Verification items for the finished model (mm, model axes). A direction names the side the tool comes from. Give positions to 0.01 mm unless a question says otherwise; leave off trailing zeros. Order: outer loops, then holes, each group sorted by start corner. A loop starts at its lowest first (then second) coordinate and runs counter-clockwise, first axis right, second up. Notation, with made-up numbers: M -26,12.25 L 3,12.25 A20 cw 3,50.25 Z; hole C 26,84 d1. An arc over 180 degrees is marked long. Answer as a JSON object with one key per item and string values.
```python
from build123d import *

# Parameters (mm, degrees)
SKETCH6_R                = 28
BOSS_EXTRUDE3_DEPTH      = 5
CUT_EXTRUDE4_DEPTH       = 1
CUT_EXTRUDE4_DEPTH_BACK  = 6
SKETCH7_8_R              = 1.5
CUT_EXTRUDE5_DEPTH       = 1
CUT_EXTRUDE5_DEPTH_BACK  = 6
SKETCH10_R               = 2
SKETCH11_R               = 2.5
CUT_EXTRUDE14_DEPTH      = 6
CUT_EXTRUDE14_DEPTH_BACK = 5
SKETCH12_R               = 9
BOSS_EXTRUDE4_DEPTH      = 4


with BuildPart() as part:
    # Sketch6 → Boss-Extrude3 (new body)
    with BuildSketch(Plane(origin=(0, 0, 0), x_dir=(1, 0, 0), z_dir=(0, 1, 0))):
        Circle(SKETCH6_R)
    extrude(amount=BOSS_EXTRUDE3_DEPTH)

    # Sketch7 → Cut-Extrude4 (cut, two sides)
    with BuildSketch(Plane(origin=(0, 5, 0), x_dir=(1, 0, 0), z_dir=(0, 1, 0))) as cut_extrude4_sk:
        with BuildLine():
            Line((12.600595793, 8.137873534), (18.900893689, 12.206810302))
            ThreePointArc((18.900893689, 12.206810302), (16.072652831, 15.745470173), (12.592900123, 18.645880684))
            Line((12.592900123, 18.645880684), (8.395266749, 12.430587123))
            ThreePointArc((8.395266749, 12.430587123), (10.715101887, 10.496980115), (12.600595793, 8.137873534))
        make_face()
        with BuildLine():
            Line((2.693946551, 14.756105583), (4.040919826, 22.134158375))
            ThreePointArc((4.040919826, 22.134158375), (0, 22.5), (-4.040919826, 22.134158375))
            Line((-4.040919826, 22.134158375), (-2.693946551, 14.756105583))
            ThreePointArc((-2.693946551, 14.756105583), (0, 15), (2.693946551, 14.756105583))
        make_face()
        with BuildLine():
            Line((-8.137873534, 12.600595793), (-12.206810302, 18.900893689))
            ThreePointArc((-12.206810302, 18.900893689), (-15.745470173, 16.072652831), (-18.645880684, 12.592900123))
            Line((-18.645880684, 12.592900123), (-12.430587123, 8.395266749))
            ThreePointArc((-12.430587123, 8.395266749), (-10.496980115, 10.715101887), (-8.137873534, 12.600595793))
        make_face()
        with BuildLine():
            Line((-14.756105583, 2.693946551), (-22.134158375, 4.040919826))
            ThreePointArc((-22.134158375, 4.040919826), (-22.5, 0), (-22.134158375, -4.040919826))
            Line((-22.134158375, -4.040919826), (-14.756105583, -2.693946551))
            ThreePointArc((-14.756105583, -2.693946551), (-15, 0), (-14.756105583, 2.693946551))
        make_face()
        with BuildLine():
            ThreePointArc((-18.900893689, -12.206810302), (-16.072652831, -15.745470173), (-12.592900123, -18.645880684))
            Line((-12.592900123, -18.645880684), (-8.395266749, -12.430587123))
            ThreePointArc((-8.395266749, -12.430587123), (-10.715101887, -10.496980115), (-12.600595793, -8.137873534))
            Line((-12.600595793, -8.137873534), (-18.900893689, -12.206810302))
        make_face()
        with BuildLine():
            ThreePointArc((-4.040919826, -22.134158375), (0, -22.5), (4.040919826, -22.134158375))
            Line((4.040919826, -22.134158375), (2.693946551, -14.756105583))
            ThreePointArc((2.693946551, -14.756105583), (0, -15), (-2.693946551, -14.756105583))
            Line((-2.693946551, -14.756105583), (-4.040919826, -22.134158375))
        make_face()
        with BuildLine():
            ThreePointArc((12.206810302, -18.900893689), (15.745470173, -16.072652831), (18.645880684, -12.592900123))
            Line((18.645880684, -12.592900123), (12.430587123, -8.395266749))
            ThreePointArc((12.430587123, -8.395266749), (10.496980115, -10.715101887), (8.137873534, -12.600595793))
            Line((8.137873534, -12.600595793), (12.206810302, -18.900893689))
        make_face()
        with BuildLine():
            ThreePointArc((22.5, 0), (22.408352945, 2.028723314), (22.134158375, 4.040919826))
            Line((22.134158375, 4.040919826), (14.756105583, 2.693946551))
            ThreePointArc((14.756105583, 2.693946551), (14.938901963, 1.352482209), (15, 0))
            ThreePointArc((15, 0), (14.938901963, -1.352482209), (14.756105583, -2.693946551))
            Line((14.756105583, -2.693946551), (22.134158375, -4.040919826))
            ThreePointArc((22.134158375, -4.040919826), (22.408352945, -2.028723314), (22.5, 0))
        make_face()
    extrude(amount=CUT_EXTRUDE4_DEPTH, mode=Mode.SUBTRACT)
    extrude(cut_extrude4_sk.sketch, amount=-CUT_EXTRUDE4_DEPTH_BACK, mode=Mode.SUBTRACT)

    # Sketch7<8> → Cut-Extrude5 (cut, two sides)
    with BuildSketch(Plane(origin=(0, 5, 0), x_dir=(1, 0, 0), z_dir=(0, 1, 0))) as cut_extrude5_sk:
        with Locations((10.5755737, 4.040919826)):
            Circle(SKETCH7_8_R)
        with Locations((10.190896389, -4.969613007)):
            Circle(SKETCH7_8_R)
        with Locations((4.476172766, 10.68433663)):
            Circle(SKETCH7_8_R)
        with Locations((3.547479586, -11.06901394)):
            Circle(SKETCH7_8_R)
        with Locations((-4.534360067, 11.06901394)):
            Circle(SKETCH7_8_R)
        with BuildLine():
            ThreePointArc((-6.876220335, -10.181386548), (-4.219994535, -11.523863304), (-6.457430859, -9.561299157))
            Line((-6.457430859, -9.561299157), (-6.876220335, -10.181386548))
        make_face()
        with Locations((-11.17777687, 4.969613007)):
            Circle(SKETCH7_8_R)
        with Locations((-11.562454181, -4.040919826)):
            Circle(SKETCH7_8_R)
    extrude(amount=CUT_EXTRUDE5_DEPTH, mode=Mode.SUBTRACT)
    extrude(cut_extrude5_sk.sketch, amount=-CUT_EXTRUDE5_DEPTH_BACK, mode=Mode.SUBTRACT)

    # Sketch10 → Cut-Revolve1 (revolve, cut)
    with BuildSketch(Plane.XY):
        with Locations((28, 2.5)):
            Circle(SKETCH10_R)
    revolve(axis=Axis((0, 40.614262211, 0), (0, -1, 0)), mode=Mode.SUBTRACT)

    # Sketch11 → Cut-Extrude14 (cut, two sides)
    with BuildSketch(Plane(origin=(0, 0, 0), x_dir=(1, 0, 0), z_dir=(0, 1, 0))) as cut_extrude14_sk:
        Circle(SKETCH11_R)
    extrude(amount=CUT_EXTRUDE14_DEPTH, mode=Mode.SUBTRACT)
    extrude(cut_extrude14_sk.sketch, amount=-CUT_EXTRUDE14_DEPTH_BACK, mode=Mode.SUBTRACT)

    # Sketch12 → Boss-Extrude4 (add)
    with BuildSketch(Plane(origin=(0, 0, 0), x_dir=(1, 0, 0), z_dir=(0, 1, 0))):
        Circle(SKETCH12_R)
        Polygon((0, 7), (-6.062177826, 3.5), (-6.062177826, -3.5), (0, -7), (6.062177826, -3.5), (6.062177826, 3.5), align=None, mode=Mode.SUBTRACT)
    extrude(amount=-BOSS_EXTRUDE4_DEPTH)


solid = part.part
```
Q1. Release check for a two-part mould opening along X. For faces 3 (the face through (25.865, 4.746, 10.724)), 4 (the face through (-3.074, -1.972, 5.226)) record: +X half, -X half, draft (parallel to the pull), parting line (faces both ways), or undercut.
Resolved:
{"face 3": "parting line", "face 4": "undercut"}
Q2. Section check A-A on y = -2.25. Record the cut outline in (x, z).
Resolved:
{"outline": "C 0,0 d18; hole M -6.06,-3.5 L 0,-7 L 6.06,-3.5 L 6.06,3.5 L 0,7 L -6.06,3.5 Z"}
Q3. Material ranges on L1, parallel to X at y = 3, z = 8.5; L2, parallel to X at y = 3, z = -17; L3, parallel to X at y = 2.25, z = -0.5, recorded low to high.
Resolved:
{"L1": "x = -24.64 to -13.16, -12.36 to 12.36, 12.59 to 24.64", "L2": "x = -19.76 to -14.74, -10.98 to -3.1, 3.1 to 11.48, 14.74 to 19.76", "L3": "x = -26.01 to -22.49, -14.99 to -2.45, 2.45 to 14.99, 22.49 to 26.01"}
Q4. Gauge pin test, flat ends, axial feed: pin 1 Ø6 at (x, z) = (3.5, 3) entering from -Y; pin 2 Ø5 at (x, z) = (4.48, -10.68) entering from -Y; pin 3 Ø1.5 at (x, z) = (-15, 11) entering from +Y; pin 4 Ø3 at (x, y) = (-17, 0.5) entering from -Z. Record the tip position at first contact, or that the pin passes through.
Resolved:
{"pin 1": "stops at y = -4", "pin 2": "stops at y = 0", "pin 3": "passes through", "pin 4": "stops at z = -23.32"}
Q5. Tool access check on faces 1 (the face through (-6.062, -2, 0)), 2 (the face through (-18.497, 2.535, 3.377)). Record the directions out of +Z, -Z, +X, -X, +Y, -Y that give a thin tool (end or side, any length) a straight path to the whole face; none if there is none.
Resolved:
{"face 1": "-Y", "face 2": "+Y, -Y"}
Q6. Section check B-B on x = -14. Count the separate pieces of the cut face and the enclosed holes in it, then the cut area to 3 significant figures.
Resolved:
{"separate pieces": "3", "enclosed holes": "0", "area": "144 mm²"}
